Design review of the part built by this model. Coordinates are the model's own, in mm. A direction names the side the tool comes from. Coordinates: 2 decimals unless noted, no trailing zeros. Loops run counter-clockwise (first coordinate to the right, second up) from the corner with the lowest first, then second, coordinate; pieces in that order, holes last. Notation, with made-up numbers: (-23.5, 55.5) - (-18.5, 55.5) arc R18 cw to (-18.5, 85.5) - close; hole circle Ø4 at (-22.75, 87). An arc over 180 degrees is marked (long way). Answer in a Markdown table with one row per item. Add a question column.
(1) For faces 4 (the face through (-12.471, 0, 1)), 5 (the face through (-4, 10, 2.896)), list the 3-axis set-ups (+Z, -Z, +X, -X, +Y, -Y) from which the entire face can be reached by the end or side of a thin tool; tool diameter is ignored.
(2) We need section B-B, the plane x = 0. Write out the cut boundary in (y, z) (3 decimals), plus the area to 3 significant figures.
(3) We need section A-A, the plane y = 0. Write out the cut boundary in (x, z).
(4) We need section D-D, the plane x = 10.75. Write out the cut boundary in (y, z).
(5) The part is to be moulded in two halves that separate along Y. For faces 1 (the face through (0, -10.795, 1)), 2 (the face through (6.76, 5.19, 14.38)), 3 (the face through (0, 10.795, 1)), say which applies: released by +Y, released by -Y, zero draft, split by the parting line, or undercut.
(6) We need section C-C, the plane z = 19.5. Write out the cut boundary in (x, y).
(7) Clearance check with flat-ended pins moving along their axes: pin 1 (2 mm diameter, centred on x = 2.5, z = 14.5, fed in from -Y); pin 2 (5 mm diameter, centred on y = -6.5, z = 25.5, fed in from +X); pin 3 (1 mm diameter, centred on y = 0.5, z = 18, fed in from +X). State where each tip first meets the part, or that it passes through.
(8) To check wall thickness, follow L1, parallel to Z at x = 8.5, y = -9; L2, parallel to Y at x = 0, z = 20.5; L3, parallel to X at y = -3, z = 20.75. State the ranges of each line that lie inside material, in increasing order. Write a range as [from, to].
from build123d import *

# Parameters (mm, degrees)
F0_R     = 10.2362
F0_R_2   = 8.51027
F1_DEPTH = 28.3591
F3_DEPTH = 2.8956
F5_D     = 17.0434
F6_SIZE  = 1.27


with BuildPart() as f1:
    # F0 (on Top) → F1 (new body)
    with BuildSketch(Plane.XY):
        Circle(F0_R)
        Circle(F0_R_2, mode=Mode.SUBTRACT)
    extrude(amount=F1_DEPTH)

    # F2 (on Top) → F3 (join)
    with BuildSketch(Plane.XY):
        with BuildLine():
            Line((-7.160593, -10.795), (7.160593, -10.795))
            ThreePointArc((7.160593, -10.795), (12.954, 0), (7.160593, 10.795))
            Line((7.160593, 10.795), (-7.160593, 10.795))
            ThreePointArc((-7.160593, 10.795), (-10.471269, 7.626181), (-12.4714, 3.502899))
            Line((-12.4714, 3.502899), (-12.4714, -3.502899))
            ThreePointArc((-12.4714, -3.502899), (-10.471269, -7.626181), (-7.160593, -10.795))
        make_face()
    extrude(amount=F3_DEPTH)

    # F5 (through all)
    with Locations(Plane(origin=(0, 0, 0), x_dir=(1, 0, 0), z_dir=(0, 0, -1))):
        with Locations((0, 0)):
            Hole(F5_D / 2)

    # F6
    f6_edges = [f1.edges().sort_by_distance(p)[0] for p in [
        (-10.2362, 0, 28.3591),
    ]]
    chamfer(f6_edges, length=F6_SIZE)


solid = f1.part
Responses:
| question | item | result |
|---|---|---|
| 1 | face 4 | +Z, -Z, -X, +Y, -Y |
| 1 | face 5 | +Z |
| 2 | outline | (-10.795, 0) - (-8.522, 0) - (-8.522, 28.359) - (-8.966, 28.359) - (-10.236, 27.089) - (-10.236, 2.896) - (-10.795, 2.896) - close; (8.522, 0) - (10.795, 0) - (10.795, 2.896) - (10.236, 2.896) - (10.236, 27.089) - (8.966, 28.359) - (8.522, 28.359) - close |
| 2 | area | 98.9 mm2 |
| 3 | outline | (-12.47, 0) - (-8.52, 0) - (-8.52, 28.36) - (-8.97, 28.36) - (-10.24, 27.09) - (-10.24, 2.9) - (-12.47, 2.9) - close; (8.52, 0) - (12.95, 0) - (12.95, 2.9) - (10.24, 2.9) - (10.24, 27.09) - (8.97, 28.36) - (8.52, 28.36) - close |
| 4 | outline | (-7.23, 0) - (7.23, 0) - (7.23, 2.9) - (-7.23, 2.9) - close |
| 5 | face 1 | released by -Y |
| 5 | face 2 | undercut |
| 5 | face 3 | released by +Y |
| 6 | outline | circle Ø20.47 at (0, 0); hole circle Ø17.04 at (0, 0) |
| 7 | pin 1 | stops at y = -10.13 |
| 7 | pin 2 | stops at x = 9.42 |
| 7 | pin 3 | stops at x = 10.24 |
| 8 | L1 | z = [0, 2.9] |
| 8 | L2 | y = [-10.24, -8.52], [8.52, 10.24] |
| 8 | L3 | x = [-9.79, -7.98], [7.98, 9.79] |
